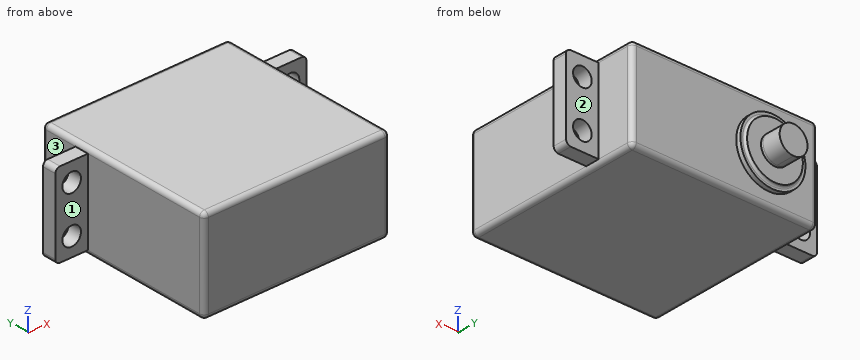
from build123d import *

# Parameters (mm, degrees)
SKETCH_1_W          = 40
SKETCH_1_H          = 39
EXTRUDE_1_DEPTH     = 20
FILLET_1_R          = 1
SKETCH_2_W          = 18
SKETCH_2_H          = 3
EXTRUDE_2_DEPTH     = 7
SKETCH_3_W          = 18
SKETCH_3_H          = 3
EXTRUDE_3_DEPTH     = 7
FILLET_8_R          = 1
FILLET_9_R          = 1
SKETCH_4_R          = 2
CUT_EXTRUDE_1_DEPTH = 7
SKETCH_5_R          = 2
CUT_EXTRUDE_2_DEPTH = 7
SKETCH_6_R          = 2
CUT_EXTRUDE_3_DEPTH = 7
SKETCH_8_R          = 2
CUT_EXTRUDE_4_DEPTH = 7
SKETCH_9_R          = 3
EXTRUDE_4_DEPTH     = 6
SKETCH_10_R         = 7
EXTRUDE_5_DEPTH     = 1
SKETCH_11_R         = 6
EXTRUDE_6_DEPTH     = 2
FILLET_11_R         = 0.5
SKETCH_12_W         = 12
SKETCH_12_H         = 0.5
CUT_EXTRUDE_6_DEPTH = 19
SKETCH_13_R         = 3
EXTRUDE_7_DEPTH     = 6


with BuildPart() as part:
    # Sketch 1 → Extrude 1 (new body)
    with BuildSketch(Plane.XY):
        with Locations((1.208791209, 10.42505216)):
            Rectangle(SKETCH_1_W, SKETCH_1_H)
    extrude(amount=EXTRUDE_1_DEPTH)

    # Fillet 1
    fillet_1_edges = [part.edges().sort_by_distance(p)[0] for p in [
        (21.208791209, 10.42505216, 20),
        (1.208791209, 29.92505216, 20),
        (-18.791208791, 10.42505216, 20),
        (1.208791209, 29.92505216, 0),
        (21.208791209, 10.42505216, 0),
        (1.208791209, -9.07494784, 0),
        (-18.791208791, 10.42505216, 0),
        (-18.791208791, 29.92505216, 10),
        (21.208791209, 29.92505216, 10),
        (21.208791209, -9.07494784, 10),
        (-18.791208791, -9.07494784, 10),
        (1.208791209, -9.07494784, 20),
    ]]
    fillet(fillet_1_edges, radius=FILLET_1_R)

    # Sketch 2 → Extrude 2 (add)
    with BuildSketch(Plane.ZY.offset(18.791208791)):
        with Locations((10, 20.42505216)):
            Rectangle(SKETCH_2_W, SKETCH_2_H)
    extrude(amount=EXTRUDE_2_DEPTH)

    # Sketch 3 → Extrude 3 (add)
    with BuildSketch(Plane(origin=(21.208791209, 0, 0), x_dir=(0, 0, -1), z_dir=(1, 0, 0))):
        with Locations((-10, 20.42505216)):
            Rectangle(SKETCH_3_W, SKETCH_3_H)
    extrude(amount=EXTRUDE_3_DEPTH)

    # Fillet 8
    fillet_8_edges = [part.edges().sort_by_distance(p)[0] for p in [
        (28.208791209, 20.42505216, 1),
    ]]
    fillet(fillet_8_edges, radius=FILLET_8_R)

    # Fillet 9
    fillet_9_edges = [part.edges().sort_by_distance(p)[0] for p in [
        (-25.791208791, 20.42505216, 19),
        (-25.791208791, 20.42505216, 1),
        (28.208791209, 20.42505216, 19),
    ]]
    fillet(fillet_9_edges, radius=FILLET_9_R)

    # Sketch 4 → Cut-Extrude 1 (cut)
    with BuildSketch(Plane(origin=(0, 21.92505216, 0), x_dir=(1, 0, 0), z_dir=(0, 1, 0))):
        with Locations(Location((-22.291208791, -5, 0), (0, 0, 180))):
            Circle(SKETCH_4_R)
    extrude(amount=-CUT_EXTRUDE_1_DEPTH, mode=Mode.SUBTRACT)

    # Sketch 5 → Cut-Extrude 2 (cut)
    with BuildSketch(Plane(origin=(0, 21.92505216, 0), x_dir=(1, 0, 0), z_dir=(0, 1, 0))):
        with Locations(Location((-22.291208791, -15, 0), (0, 0, 180))):
            Circle(SKETCH_5_R)
    extrude(amount=-CUT_EXTRUDE_2_DEPTH, mode=Mode.SUBTRACT)

    # Sketch 6 → Cut-Extrude 3 (cut)
    with BuildSketch(Plane(origin=(0, 21.92505216, 0), x_dir=(1, 0, 0), z_dir=(0, 1, 0))):
        with Locations(Location((24.708791209, -5, 0), (0, 0, 180))):
            Circle(SKETCH_6_R)
    extrude(amount=-CUT_EXTRUDE_3_DEPTH, mode=Mode.SUBTRACT)

    # Sketch 8 → Cut-Extrude 4 (cut)
    with BuildSketch(Plane(origin=(0, 21.92505216, 0), x_dir=(1, 0, 0), z_dir=(0, 1, 0))):
        with Locations(Location((24.708791209, -15, 0), (0, 0, 180))):
            Circle(SKETCH_8_R)
    extrude(amount=-CUT_EXTRUDE_4_DEPTH, mode=Mode.SUBTRACT)

    # Sketch 9 → Extrude 4 (add)
    with BuildSketch(Plane(origin=(0, 29.92505216, 0), x_dir=(1, 0, 0), z_dir=(0, 1, 0))):
        with Locations(Location((-8.291208791, -10, 0), (0, 0, 90))):
            Circle(SKETCH_9_R)
    extrude(amount=EXTRUDE_4_DEPTH)

    # Sketch 10 → Extrude 5 (add)
    with BuildSketch(Plane(origin=(0, 29.92505216, 0), x_dir=(1, 0, 0), z_dir=(0, 1, 0))):
        with Locations(Location((-8.291208791, -10, 0), (0, 0, 90))):
            Circle(SKETCH_10_R)
    extrude(amount=EXTRUDE_5_DEPTH)

    # Sketch 11 → Extrude 6 (add)
    with BuildSketch(Plane(origin=(0, 29.92505216, 0), x_dir=(1, 0, 0), z_dir=(0, 1, 0))):
        with Locations(Location((-8.291208791, -10, 0), (0, 0, 270))):
            Circle(SKETCH_11_R)
    extrude(amount=EXTRUDE_6_DEPTH)

    # Fillet 11
    fillet_11_edges = [part.edges().sort_by_distance(p)[0] for p in [
        (-8.291208791, 30.92505216, 4),
        (-8.291208791, 31.92505216, 4),
    ]]
    fillet(fillet_11_edges, radius=FILLET_11_R - 0.0001)  # a hair under: the kernel refuses the full size

    # Sketch 12 → Cut-Extrude 6 (cut)
    with BuildSketch(Plane.XY.offset(20)):
        with Locations((-8.291208791, 31.67505216)):
            Rectangle(SKETCH_12_W, SKETCH_12_H)
    extrude(amount=-CUT_EXTRUDE_6_DEPTH, mode=Mode.SUBTRACT)


with BuildPart() as cut_extrude_6_piece_1:
    # of the separate pieces the step leaves, piece 1, a body of its own (cut_extrude_6_pieces)
    add(part.part.solids().sort_by_distance((-8.291208791, 30.92505216, 16.4999))[0])



with BuildPart() as cut_extrude_6_piece_2:
    # of the separate pieces the step leaves, piece 2, a body of its own (cut_extrude_6_pieces)
    add(part.part.solids().sort_by_distance((-8.291208791, 31.92505216, 7))[0])


with BuildPart() as cut_extrude_6_piece_1_1:
    add(cut_extrude_6_piece_1.part)

    add(cut_extrude_6_piece_2.part)  # Extrude 7 merges Cut-Extrude 6 piece 2
    # Sketch 13 → Extrude 7 (add)
    with BuildSketch(Plane(origin=(0, 35.92505216, 0), x_dir=(1, 0, 0), z_dir=(0, 1, 0))):
        with Locations(Location((-8.291208791, -10, 0), (0, 0, 270))):
            Circle(SKETCH_13_R)
    extrude(amount=-EXTRUDE_7_DEPTH)


solid = cut_extrude_6_piece_1_1.part
Here's how the part is built. I have some questions about the finished solid (model axes, mm). Face numbers are marked on the shaded views. A direction names the side the tool comes from. Give positions to 0.01 mm unless a question says otherwise; leave off trailing zeros. Loops run counter-clockwise (first coordinate to the right, second up) from the corner with the lowest first, then second, coordinate; pieces in that order, holes last. Notation, with made-up numbers: (40, 0.5) -> (82, 0.5) arc R19 ccw to (82, 6.5) -> close; hole circle Ø8 at (26.25, -35.75). An arc over 180 degrees is marked (long way). Answer as a JSON object with one key per item and string values. Group by question number.
Item 1: Imagine slicing it at A-A on y = 21. Write out the boundary of the cut face in (x, z), then the cut area to 3 significant figures.
Item 2: Imagine slicing it at B-B on x = -16.5. Write out the boundary of the cut face in (y, z), then the cut area to 3 significant figures.
Item 3: Imagine slicing it at D-D on z = 5. Give the number of separate pieces and of enclosed holes in the cut face, then the cut area to 3 significant figures.
Item 4: On a 3-axis mill with a long thin cutter (end or side, diameter ignored), from which of +Z, -Z, +X, -X, +Y, -Y can I reach the whole of each face in a straight line? I mean the marked faces 1, 2 and 3. Say none if no direction works.
Item 5: Will these pins go through, and if not, where does the flat tip stop? pin 1 (6.5 mm diameter, centred on x = 24.71, z = 5, fed in from +Y); pin 2 (10 mm diameter, centred on x = 0, z = 10, fed in from +Y); pin 3 (10 mm diameter, centred on x = 8.5, z = 2.5, fed in from +Y); pin 4 (3.5 mm diameter, centred on x = 24.71, z = 15, fed in from -Y).
Item 6: I need wall thicknesses on L1, parallel to Y at x = -16, z = 8.75; L2, parallel to X at y = 7, z = 4.25; L3, parallel to Y at x = 22.5, z = 16.75. Which ranges of each line are inside material? Lowest first, please.
Answer list:
{
 "1": {"outline": "(-25.79, 2) arc R1 ccw to (-24.79, 1) -> (-18.79, 1) arc R1 ccw to (-17.79, 0) -> (20.21, 0) arc R1 ccw to (21.21, 1) -> (27.21, 1) arc R1 ccw to (28.21, 2) -> (28.21, 18) arc R1 ccw to (27.21, 19) -> (21.21, 19) arc R1 ccw to (20.21, 20) -> (-17.79, 20) arc R1 ccw to (-18.79, 19) -> (-24.79, 19) arc R1 ccw to (-25.79, 18) -> close; hole circle Ø4 at (-22.29, 5); hole circle Ø4 at (-22.29, 15); hole circle Ø4 at (24.71, 5); hole circle Ø4 at (24.71, 15)", "area": "1,000 mm2"},
 "2": {"outline": "(-9.07, 1) arc R1 ccw to (-8.07, 0) -> (28.93, 0) arc R1 ccw to (29.93, 1) -> (29.93, 19) arc R1 ccw to (28.93, 20) -> (-8.07, 20) arc R1 ccw to (-9.07, 19) -> close", "area": "779 mm2"},
 "3": {"separate pieces": "3", "enclosed holes": "0", "area": "1,590 mm2"},
 "4": {"face 1": "+Z, -Z, -X, -Y", "face 2": "+Z, -Z, +X, +Y", "face 3": "+Z, -Z, -X, +Y"},
 "5": {"pin 1": "stops at y = 21.93", "pin 2": "stops at y = 31.43", "pin 3": "stops at y = 29.93", "pin 4": "passes through"},
 "6": {"L1": "y = -9.07 to 29.93", "L2": "x = -18.79 to 21.21", "L3": "y = 18.93 to 21.93"}
}
